For this review, take the finished solid that the model builds, in its own axes (mm). A direction names the side the tool comes from. Give positions to 0.01 mm unless a question says otherwise; leave off trailing zeros. Order: outer loops, then holes, each group sorted by start corner. A loop starts at its lowest first (then second) coordinate and runs counter-clockwise, first axis right, second up. Notation, with made-up numbers: (-29, 10) -> (-14, 10) arc R19 ccw to (-14, 15) -> close; hole circle Ø2 at (22.5, 86.5). An arc over 180 degrees is marked (long way). One line per item, written item: value. Start each with the question number.
from build123d import *

# Parameters (mm, degrees)
SKETCH1_R           = 8.425
BOSS_EXTRUDE1_DEPTH = 11
SKETCH3_R           = 8.425
BOSS_EXTRUDE2_DEPTH = 11
SKETCH4_R           = 4.25
CUT_EXTRUDE1_DEPTH  = 27.096192251
BOSS_EXTRUDE3_DEPTH = 22
CHAMFER1_SIZE       = 1
SKETCH6_R           = 6.5
BOSS_EXTRUDE4_DEPTH = 9
BOSS_EXTRUDE5_DEPTH = 8
SKETCH10_R          = 1.104065367
CUT_EXTRUDE2_DEPTH  = 35.029564352


with BuildPart() as part:
    # Sketch1 → Boss-Extrude1 (new body)
    with BuildSketch(Plane(origin=(0, 0, 0), x_dir=(1, 0, 0), z_dir=(0, 1, 0))):
        with Locations(Location((0, 0, 0), (0, 0, 270))):
            Circle(SKETCH1_R)
    extrude(amount=BOSS_EXTRUDE1_DEPTH)

    # Sketch3 → Boss-Extrude2 (add)
    with BuildSketch(Plane.XZ):
        with Locations(Location((1.5, 1.5, 0), (0, 0, 142.232408159))):
            Circle(SKETCH3_R)
    extrude(amount=BOSS_EXTRUDE2_DEPTH)

    # Sketch4 → Cut-Extrude1 (cut, through all)
    with BuildSketch(Plane.XZ.offset(11)):
        with Locations(Location((1.5, 0, 0), (0, 0, 270))):
            Circle(SKETCH4_R)
    extrude(amount=-CUT_EXTRUDE1_DEPTH, mode=Mode.SUBTRACT)

    # Sketch5 → Boss-Extrude3 (add)
    with BuildSketch(Plane.XZ.offset(11)):
        with BuildLine():
            Line((-2.05, 2.336664289), (-2.05, -2.336664289))
            ThreePointArc((-2.05, -2.336664289), (-2.75, 0), (-2.05, 2.336664289))
        make_face()
    extrude(amount=-BOSS_EXTRUDE3_DEPTH)

    # Chamfer1
    chamfer1_edges = [part.edges().sort_by_distance(p)[0] for p in [
        (8.159975677, -11, -3.659975677),
    ]]
    chamfer(chamfer1_edges, length=CHAMFER1_SIZE)

    # Sketch6 → Boss-Extrude4 (add)
    with BuildSketch(Plane(origin=(0, 11, 0), x_dir=(1, 0, 0), z_dir=(0, 1, 0))):
        with Locations(Location((1.5, 0, 0), (0, 0, 270))):
            Circle(SKETCH6_R)
        with BuildLine():
            Line((-2.05, 2.336664289), (-2.05, -2.336664289))
            ThreePointArc((-2.05, -2.336664289), (5.75, 0), (-2.05, 2.336664289))
        make_face(mode=Mode.SUBTRACT)
    extrude(amount=BOSS_EXTRUDE4_DEPTH)

    # Sketch7 → Boss-Extrude5 (add)
    with BuildSketch(Plane.XZ.offset(11)):
        with BuildLine():
            Line((-2.05, -2.336664289), (-2.05, 2.336664289))
            ThreePointArc((-2.05, 2.336664289), (5.75, 0), (-2.05, -2.336664289))
        make_face()
    extrude(amount=-BOSS_EXTRUDE5_DEPTH)

    # Sketch10 → Cut-Extrude2 (cut, through all)
    with BuildSketch(Plane.XZ.offset(11)):
        with Locations(Location((1.534537663, 0, 0), (0, 0, 270))):
            Circle(SKETCH10_R)
    extrude(amount=-CUT_EXTRUDE2_DEPTH, mode=Mode.SUBTRACT)


solid = part.part
Q1. For faces 5 (the cylindrical face through (7.981, -4.93, 6.883)), 6 (the flat face through (-3, 20, 0)), 7 (the flat face through (3, -3, 0)), list the 3-axis set-ups (+Z, -Z, +X, -X, +Y, -Y) from which the entire face can be reached by the end or side of a thin tool; tool diameter is ignored.
Q2. Mouldability with a two-part tool opening along X and no side actions: class faces 1 (the cylindrical face through (2, -7, -1)), 2 (the flat face through (-2.05, 8, 0)), 3 (the flat face through (6.1, 0, 6.3)), 4 (the cylindrical face through (-2.455, 15.437, -5.158)) as pulls with the +X half, pulls with the -X half, needs draft (parallel to the pull), parting line crosses it, or undercut.
Q3. For line 1 along X through (y, z) = (5.5, 0) (3 decimals); line 2 along X through (y, z) = (13.5, 0); line 3 along Z through (x, y) = (1.5, -9.5) (3 decimals), list the stretches that pass through material, from the lowest coordinate up.
Q4. For pin 1 Ø2.5 at (y, z) = (13.5, 1) entering from +X; pin 2 Ø5 at (x, y) = (-3, 14.5) entering from +Z; pin 3 Ø8 at (y, z) = (13.5, 6) entering from -X, all flat-tipped, find the tip position at first contact; note any pin that passes through.
Q5. Take a section at B-B (y = 7.5). State the section outline as (x, z) points (3 decimals).
Q6. Take a section at C-C (y = -7). State the section outline as (x, z) points (3 decimals).
Answers below:
1. face 5: -Y
1. face 6: +Z, -Z, +X, -X, +Y
1. face 7: +Y
2. face 1: undercut
2. face 2: undercut
2. face 3: needs draft
2. face 4: parting line crosses it
3. line 1: x = -8.425 to -2.05, 5.75 to 8.425
3. line 2: x = -5 to -2.05, 5.75 to 8
3. line 3: z = -6.925 to -1.104, 1.104 to 9.925
4. pin 1: stops at x = 8
4. pin 2: stops at z = 6.18
4. pin 3: stops at x = -7.92
5. outline: circle Ø16.85 at (0, 0); hole (-2.05, -2.337) arc R4.25 ccw (long way) to (-2.05, 2.337) -> close
6. outline: circle Ø16.85 at (1.5, 1.5); hole circle Ø2.208 at (1.535, 0)
